Check sheet for the modelled part. Datum: model origin and axes. Units: mm. Coordinates: 2 decimals unless noted, no trailing zeros. Write each loop counter-clockwise with the first axis right and the second up, starting at its lowest first coordinate (ties: lowest second). Pieces come first, ordered by that corner, then holes. Notation, with made-up numbers: (-7, -39) -> (10, -39) arc R12 ccw to (10, -27) -> close; hole circle Ø3 at (28.5, 24.25). An arc over 180 degrees is marked (long way). One line per item, written item: value. Start each with the question number.
1) Sectioned sample at B-B on z = 0. Enter the section's corners in (x, y).
2) Scan lines: line 1 along Y through (x, z) = (4.05, 0); line 2 along Z through (x, y) = (0, 34.5). Record each from-to range of solid material in increasing order. Write a range as [from, to].
3) Gauge pin test, flat ends, axial feed: P1, Ø2.5, axis at y = 115, z = 0, coming from the +X side; P2, Ø5, axis at y = 87, z = 2.5, coming from the +X side; P3, Ø3, axis at x = -2, y = 87, coming from the -Z side. Record the tip position at first contact, or that the pin passes through.
4) Draft check along X on faces 1 (the flat face through (-3, 0, 3)), 2 (the cylindrical face through (4.292, 59.16, -1.352)), 3 (the cylindrical face through (-0.867, 59.16, 3.905)). Enter one of: +X half, -X half, draft (parallel to the pull), parting line (faces both ways), or undercut.
5) Sectioned sample at A-A on x = 0. Enter the section's corners in (y, z), plus the area to 3 significant figures.
6) Sectioned sample at C-C on y = 16.5. Enter the section's corners in (x, z), plus the area to 3 significant figures.
```python
from build123d import *

# Parameters (mm, degrees)
CROQUIS1_R                 = 4.5
CROQUIS1_R_2               = 4
SALIENTE_EXTRUIR1_DEPTH    = 120
CROQUIS2_R                 = 1.5
CORTAR_EXTRUIR1_DEPTH      = 5.5
CORTAR_EXTRUIR1_DEPTH_BACK = 5.5


with BuildPart() as part:
    # Croquis1 → Saliente-Extruir1 (new body)
    with BuildSketch(Plane(origin=(0, 0, 0), x_dir=(1, 0, 0), z_dir=(0, 1, 0))):
        Circle(CROQUIS1_R)
        Circle(CROQUIS1_R_2, mode=Mode.SUBTRACT)
    extrude(amount=SALIENTE_EXTRUIR1_DEPTH)

    # Croquis2 → Cortar-Extruir1 (cut, two sides)
    with BuildSketch(Plane(origin=(0, 0, 0), x_dir=(0, 0, -1), z_dir=(1, 0, 0))) as cortar_extruir1_sk:
        with Locations((0, 115)):
            Circle(CROQUIS2_R)
        with Locations((0, 5)):
            Circle(CROQUIS2_R)
    extrude(amount=CORTAR_EXTRUIR1_DEPTH, mode=Mode.SUBTRACT)
    extrude(cortar_extruir1_sk.sketch, amount=-CORTAR_EXTRUIR1_DEPTH_BACK, mode=Mode.SUBTRACT)


solid = part.part
```
Answers:
1. outline: (-4.5, 0) -> (-4, 0) -> (-4, 3.5) -> (-4.5, 3.5) -> close; (-4.5, 6.5) -> (-4, 6.5) -> (-4, 113.5) -> (-4.5, 113.5) -> close; (-4.5, 116.5) -> (-4, 116.5) -> (-4, 120) -> (-4.5, 120) -> close; (4, 0) -> (4.5, 0) -> (4.5, 3.5) -> (4, 3.5) -> close; (4, 6.5) -> (4.5, 6.5) -> (4.5, 113.5) -> (4, 113.5) -> close; (4, 116.5) -> (4.5, 116.5) -> (4.5, 120) -> (4, 120) -> close
2. line 1: y = [0, 3.5], [6.5, 113.5], [116.5, 120]
2. line 2: z = [-4.5, -4], [4, 4.5]
3. P1: passes through
3. P2: stops at x = 4.5
3. P3: stops at z = -4.47
4. face 1: draft
4. face 2: parting line
4. face 3: undercut
5. outline: (0, -4.5) -> (120, -4.5) -> (120, -4) -> (0, -4) -> close; (0, 4) -> (120, 4) -> (120, 4.5) -> (0, 4.5) -> close
5. area: 120 mm2
6. outline: circle Ø9 at (0, 0); hole circle Ø8 at (0, 0)
6. area: 13.4 mm2
